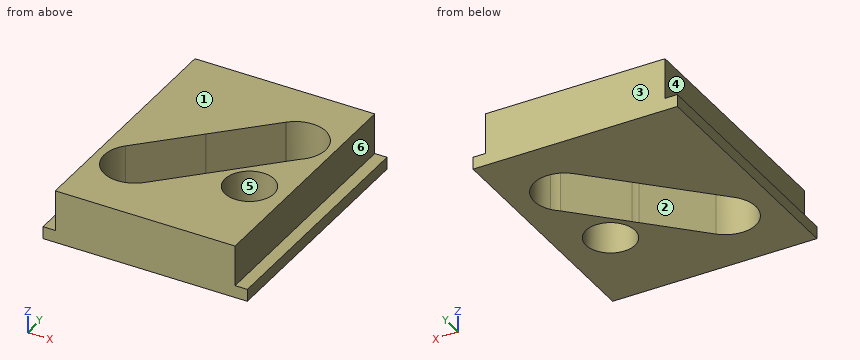
```python
from build123d import *

# Parameters (mm, degrees)
F0_W     = 50
F0_H     = 60
F0_R     = 6
F1_DEPTH = 13
F2_W     = 3
F2_H     = 60
F3_DEPTH = 10


with BuildPart() as f1:
    # F0 (on Top) → F1 (new body)
    with BuildSketch(Plane.XY):
        Rectangle(F0_W, F0_H)
        with Locations((13, -8)):
            Circle(F0_R, mode=Mode.SUBTRACT)
        with BuildLine():
            ThreePointArc((5.824037, -4.725525), (5.314884, -5.291693), (4.750949, -5.803317))
            Line((4.750949, -5.803317), (-7.185116, -17.791693))
            ThreePointArc((-7.185116, -17.791693), (-17.79758, -17.809016), (-17.803141, -7.196539))
            Line((-17.803141, -7.196539), (-5.365959, 5.239893))
            ThreePointArc((-5.365959, 5.239893), (-5.303141, 5.303461), (-5.23957, 5.366275))
            Line((-5.23957, 5.366275), (7.108243, 17.713344))
            ThreePointArc((7.108243, 17.713344), (7.196859, 17.803461), (7.286981, 17.892071))
            ThreePointArc((7.286981, 17.892071), (17.450432, 18.134113), (18.517909, 8.023979))
            ThreePointArc((18.517909, 8.023979), (17.814884, 7.208307), (17.002295, 6.501722))
            Line((17.002295, 6.501722), (5.824037, -4.725525))
        make_face(mode=Mode.SUBTRACT)
    extrude(amount=F1_DEPTH)

    # F2 (on face) → F3 (cut)
    with BuildSketch(Plane.XY.offset(13)):
        with Locations((-23.5, 0)):
            Rectangle(F2_W, F2_H)
        with Locations((23.5, 0)):
            Rectangle(F2_W, F2_H)
    extrude(amount=-F3_DEPTH, mode=Mode.SUBTRACT)


solid = f1.part
```
Check sheet for the modelled part. Datum: model origin and axes. Units: mm. Face numbers are marked on the shaded views. A direction names the side the tool comes from. Give positions to 0.01 mm unless a question says otherwise; leave off trailing zeros. Order: outer loops, then holes, each group sorted by start corner. A loop starts at its lowest first (then second) coordinate and runs counter-clockwise, first axis right, second up. Notation, with made-up numbers: M -25,61.25 L -9,61.25 A29 ccw -9,92.25 Z; hole C 47.25,44 d9. An arc over 180 degrees is marked long. Answer in a Markdown table with one row per item. Add a question column.
Q1. Sectioned sample at A-A, the plane z = 8.25. Record the boundary of the cut face in (x, y).
Q2. Gauge pin test, flat ends, axial feed: pin 1 Ø1.5 at (y, z) = (-1, 11) entering from +X; pin 2 Ø1.5 at (x, y) = (-23.5, 4) entering from +Z. Record the tip position at first contact, or that the pin passes through.
Q3. Sectioned sample at D-D, the plane y = -12.5. Record the boundary of the cut face in (x, z).
Q4. Sectioned sample at C-C, the plane x = -12.5. Record the boundary of the cut face in (y, z).
Q5. Release check for a two-part mould opening along X. For the marked faces 3, 4, 5 and 6 record: released by +X, released by -X, zero draft, split by the parting line, or undercut.
Q6. Sectioned sample at B-B, the plane y = -19. Record the boundary of the cut face in (x, z).
Q7. Access from +Z, -Z, +X, -X, +Y, -Y to the whole of each face (thin tool, end or side, straight path). Record for the marked faces 1 and 2.
Q8. Thickness scan on L1, parallel to Y at x = 13, z = 3.25; L2, parallel to X at y = -4, z = 6; L3, parallel to X at y = 9, z = 2.5. Record the ranges inside material, lowest first.
Verdict:
| question | item | result |
|---|---|---|
| 1 | outline | M -22,-30 L 22,-30 L 22,30 L -22,30 Z; hole M -17.8,-7.2 A7.5 ccw -7.19,-17.79 L 4.75,-5.8 A7.5 ccw 5.82,-4.73 L 17,6.5 A7.5 ccw 18.52,8.02 A7.5 ccw 7.29,17.89 A7.5 ccw 7.11,17.71 L -5.24,5.37 A7.5 ccw -5.37,5.24 Z; hole C 13,-8 d12 |
| 2 | pin 1 | x = 22 |
| 2 | pin 2 | z = 3 |
| 3 | outline | M -25,0 L -20,0 L -20,13 L -22,13 L -22,3 L -25,3 Z; M -1.92,0 L 9.03,0 L 9.03,13 L -1.92,13 Z; M 16.97,0 L 25,0 L 25,3 L 22,3 L 22,13 L 16.97,13 Z |
| 4 | outline | M -30,0 L -20,0 L -20,13 L -30,13 Z; M -1.89,0 L 30,0 L 30,13 L -1.89,13 Z |
| 5 | face 3 | zero draft |
| 5 | face 4 | released by -X |
| 5 | face 5 | undercut |
| 5 | face 6 | released by +X |
| 6 | outline | M -25,0 L -16.24,0 L -16.24,13 L -22,13 L -22,3 L -25,3 Z; M -8.76,0 L 25,0 L 25,3 L 22,3 L 22,13 L -8.76,13 Z |
| 7 | face 1 | +Z, +X, -X, +Y, -Y |
| 7 | face 2 | +Z, -Z |
| 8 | L1 | -30 to -14, -2 to 2.48, 19.98 to 30 |
| 8 | L2 | -22 to -14.61, 6.55 to 8.53, 17.47 to 22 |
| 8 | L3 | -25 to -1.61, 19.13 to 25 |
